Verification items for this drawing (mm, ordinates from the low corner). A direction names the side the tool comes from. Coordinates: 2 decimals unless noted, no trailing zeros. Order: outer loops, then holes, each group sorted by start corner. A loop starts at its lowest first (then second) coordinate and runs counter-clockwise, first axis right, second up.
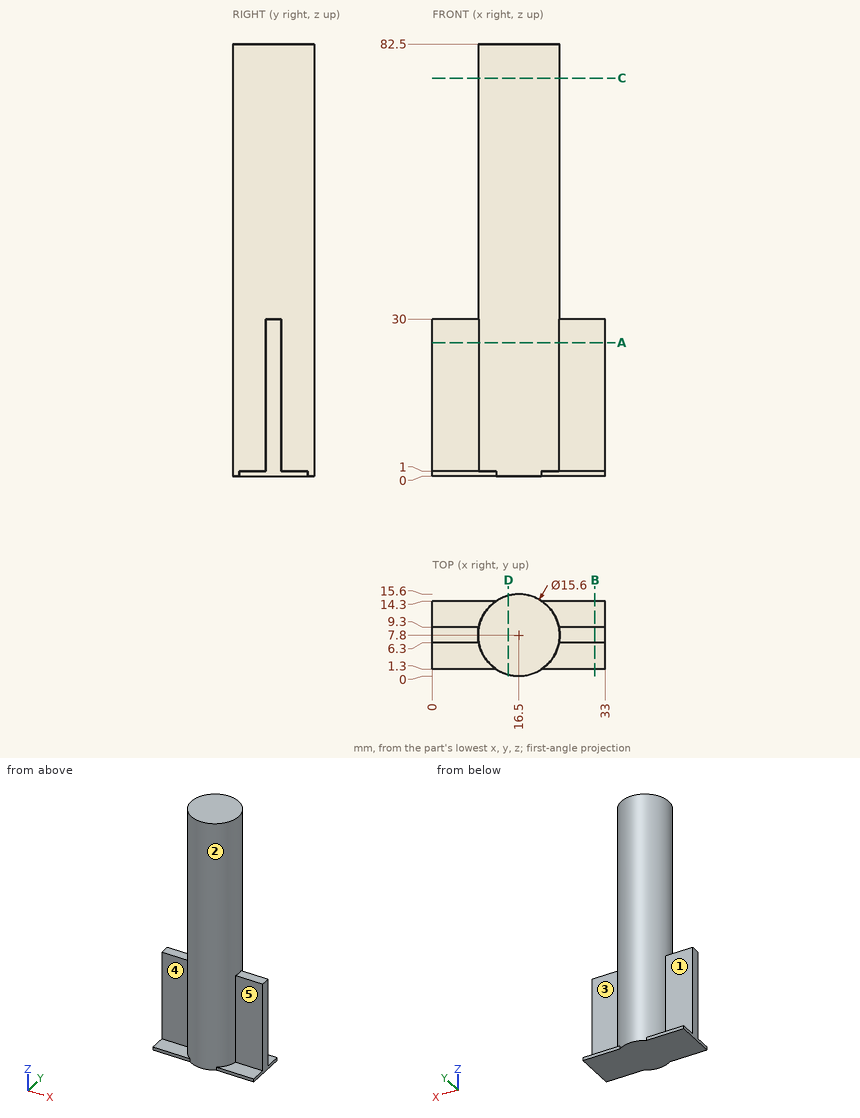
(1) Tool access check on the marked faces 1, 2, 3, 4 and 5. Record the directions out of +Z, -Z, +X, -X, +Y, -Y that give a thin tool (end or side, any length) a straight path to the whole face; none if there is none.
Filled in:
face 1: +Z, -X, +Y
face 2: +Z
face 3: +Z, +X, +Y
face 4: +Z, -X, -Y
face 5: +Z, +X, -Y
(2) Thickness scan on probe 1 along Z at (x, y) = (28.5, 7.5); probe 2 along Y at (x, z) = (5, 20); probe 3 along Z at (x, y) = (3, 2.75). Record the ranges inside material, lowest first.
Filled in:
probe 1: z = 0 to 30
probe 2: y = 6.3 to 9.3
probe 3: z = 0 to 1
(3) Cross-section at C-C (z = 76). Enter the section's corners in (x, y).
Filled in:
outline: circle Ø15.6 at (16.5, 7.8)
(4) Cross-section at B-B (x = 31). Enter the section's corners in (y, z), and give its area (3 significant figures).
Filled in:
outline: (1.3, 0) - (14.3, 0) - (14.3, 1) - (9.3, 1) - (9.3, 30) - (6.3, 30) - (6.3, 1) - (1.3, 1) - close
area: 100 mm2
(5) Go/stop test with flat-tipped pins: P1, Ø0.5, axis at x = 29, z = 0.5, coming from the -Y side; P2, Ø4, axis at x = 7.5, y = 12.5, coming from the +Z side; P3, Ø5, axis at x = 27.5, y = 8.5, coming from the +Z side. Record where each tip stops, or that it passes through.
Filled in:
P1: stops at y = 1.3
P2: stops at z = 1
P3: stops at z = 30
(6) Cross-section at D-D (x = 14.5). Enter the section's corners in (y, z).
Filled in:
outline: (0.26, 0) - (15.34, 0) - (15.34, 82.5) - (0.26, 82.5) - close
(7) Cross-section at A-A (z = 25.5). Enter the section's corners in (x, y), and give its area (3 significant figures).
Filled in:
outline: (0, 6.3) - (8.85, 6.3) arc R7.8 ccw to (24.15, 6.3) - (33, 6.3) - (33, 9.3) - (24.15, 9.3) arc R7.8 ccw to (8.85, 9.3) - (0, 9.3) - close
area: 244 mm2
